```python
from build123d import *

# Parameters (mm, degrees)
SKETCH_1_W          = 300
SKETCH_1_H          = 145
EXTRUDE_1_DEPTH     = 60
SHELL_1_T           = -6
SKETCH_2_R          = 2.55
CUT_EXTRUDE_1_DEPTH = 176.134947969
SKETCH_3_W          = 300
SKETCH_3_H          = 145
CUT_EXTRUDE_2_DEPTH = 176.134947969
SKETCH_4_R          = 1.6
CUT_EXTRUDE_3_DEPTH = 167.71007768
SKETCH_5_R          = 2.95
CUT_EXTRUDE_5_DEPTH = 3


with BuildPart() as part:
    # ｽｹｯﾁ1 → ﾎﾞｽ - 押し出し1 (new body)
    with BuildSketch(Plane(origin=(0, 0, 0), x_dir=(1, 0, 0), z_dir=(0, 1, 0))):
        Rectangle(SKETCH_1_W, SKETCH_1_H)
    extrude(amount=EXTRUDE_1_DEPTH)

    # ｼｪﾙ1
    shell_1_openings = [part.faces().sort_by_distance(p)[0] for p in [
        (0, 60, 0),
    ]]
    offset(amount=SHELL_1_T, openings=shell_1_openings, kind=Kind.INTERSECTION)

    # ｽｹｯﾁ2 → ｶｯﾄ - 押し出し1 (cut, through all)
    with BuildSketch(Plane(origin=(0, 6, 0), x_dir=(1, 0, 0), z_dir=(0, 1, 0))):
        with Locations(Location((140, 60, 0), (0, 0, 270))):
            Circle(SKETCH_2_R)
        with Locations(Location((140, -60, 0), (0, 0, 90))):
            Circle(SKETCH_2_R)
        with Locations(Location((-22.5, -60, 0), (0, 0, 270))):
            Circle(SKETCH_2_R)
        with Locations(Location((-22.5, 60, 0), (0, 0, 90))):
            Circle(SKETCH_2_R)
    extrude(amount=-CUT_EXTRUDE_1_DEPTH, mode=Mode.SUBTRACT)

    # ｽｹｯﾁ3 → ｶｯﾄ - 押し出し2 (cut, through all)
    with BuildSketch(Plane(origin=(0, 6, 0), x_dir=(1, 0, 0), z_dir=(0, 1, 0))):
        Rectangle(SKETCH_3_W, SKETCH_3_H)
    extrude(amount=CUT_EXTRUDE_2_DEPTH, mode=Mode.SUBTRACT)

    # ｽｹｯﾁ4 → ｶｯﾄ - 押し出し3 (cut, through all)
    with BuildSketch(Plane.XZ):
        with Locations(Location((147, 0, 0), (0, 0, 270))):
            Circle(SKETCH_4_R)
        with Locations(Location((147, 40, 0), (0, 0, 270))):
            Circle(SKETCH_4_R)
        with Locations(Location((147, -40, 0), (0, 0, 90))):
            Circle(SKETCH_4_R)
        with Locations(Location((-147, -40, 0), (0, 0, 270))):
            Circle(SKETCH_4_R)
        with Locations(Location((-147, 0, 0), (0, 0, 90))):
            Circle(SKETCH_4_R)
        with Locations(Location((-147, 40, 0), (0, 0, 90))):
            Circle(SKETCH_4_R)
        with Locations(Location((0, 69.5, 0), (0, 0, 270))):
            Circle(SKETCH_4_R)
        with Locations(Location((-80, 69.5, 0), (0, 0, 270))):
            Circle(SKETCH_4_R)
        with Locations(Location((80, 69.5, 0), (0, 0, 90))):
            Circle(SKETCH_4_R)
        with Locations(Location((80, -69.5, 0), (0, 0, 270))):
            Circle(SKETCH_4_R)
        with Locations(Location((0, -69.5, 0), (0, 0, 90))):
            Circle(SKETCH_4_R)
        with Locations(Location((-80, -69.5, 0), (0, 0, 90))):
            Circle(SKETCH_4_R)
    extrude(amount=-CUT_EXTRUDE_3_DEPTH, mode=Mode.SUBTRACT)

    # ｽｹｯﾁ5 → ｶｯﾄ - 押し出し5 (cut)
    with BuildSketch(Plane(origin=(0, 6, 0), x_dir=(1, 0, 0), z_dir=(0, 1, 0))):
        with Locations(Location((147, -40, 0), (0, 0, 270))):
            Circle(SKETCH_5_R)
        with Locations(Location((147, 0, 0), (0, 0, 270))):
            Circle(SKETCH_5_R)
        with Locations(Location((147, 40, 0), (0, 0, 270))):
            Circle(SKETCH_5_R)
        with Locations(Location((80, 69.5, 0), (0, 0, 270))):
            Circle(SKETCH_5_R)
        with Locations(Location((0, 69.5, 0), (0, 0, 270))):
            Circle(SKETCH_5_R)
        with Locations(Location((-80, 69.5, 0), (0, 0, 270))):
            Circle(SKETCH_5_R)
        with Locations(Location((-147, 40, 0), (0, 0, 270))):
            Circle(SKETCH_5_R)
        with Locations(Location((-147, 0, 0), (0, 0, 270))):
            Circle(SKETCH_5_R)
        with Locations(Location((-147, -40, 0), (0, 0, 270))):
            Circle(SKETCH_5_R)
        with Locations(Location((80, -69.5, 0), (0, 0, 270))):
            Circle(SKETCH_5_R)
        with Locations(Location((0, -69.5, 0), (0, 0, 270))):
            Circle(SKETCH_5_R)
        with Locations(Location((-80, -69.5, 0), (0, 0, 270))):
            Circle(SKETCH_5_R)
    extrude(amount=-CUT_EXTRUDE_5_DEPTH, mode=Mode.SUBTRACT)


solid = part.part
```
Model file for the job. Use its own axes, mm. A direction names the side the tool comes from. Coordinates: 2 decimals unless noted, no trailing zeros. Answer as a JSON object with one key per item and string values.
Q1. Pull direction Z, two halves, no side cores. Call faces 3 (the cylindrical face through (142.53, 3.04, -60.33)), 4 (the flat face through (-2, 0, -1)), 5 (the flat face through (-2, 3, 72.5)): released by +Z, released by -Z, zero draft, split by the parting line, or undercut.
Report:
{"face 3": "undercut", "face 4": "zero draft", "face 5": "released by +Z"}
Q2. 3-axis set-ups, long thin cutter, end or side, ignore diameter. For faces 1 (the flat face through (-150, 3, 1)), 2 (the flat face through (79, 3, 71)): which of +Z, -Z, +X, -X, +Y, -Y reach the whole face in a straight line?
Report:
{"face 1": "+Z, -Z, -X, +Y, -Y", "face 2": "+Y"}
Q3. Flat gauge pin, fed straight in: P1, Ø5.5, axis at x = -147, z = 40, coming from the +Y side. Where does the tip first touch, or does it go through?
Report:
{"P1": "stops at y = 3"}
Q4. Probe probe 1 along Z at (x, y) = (-22, 4.5); probe 2 along Z at (x, y) = (-147, 2.25); probe 3 along Z at (x, y) = (-80, 2.05). List the from-to ranges inside material, lowest first.
Report:
{"probe 1": "z = -72.5 to -62.5, -57.5 to 57.5, 62.5 to 72.5", "probe 2": "z = -72.5 to -41.6, -38.4 to -1.6, 1.6 to 38.4, 41.6 to 72.5", "probe 3": "z = -72.5 to -71.1, -67.9 to 67.9, 71.1 to 72.5"}
